Work out the finished part from the listing and answer in its coordinate system (mm). Face numbers are marked on the shaded views. A direction names the side the tool comes from. Round coordinates to 2 decimals unless told otherwise and drop trailing zeros. Loops run counter-clockwise (first coordinate to the right, second up) from the corner with the lowest first, then second, coordinate; pieces in that order, holes last.
Autodesk Inventor part; units mm, degrees
ref_plane "YZ Plane" through (0, 0, 0) normal (1, 0, 0) x (0, 1, 0)
ref_plane "XZ Plane" through (0, 0, 0) normal (0, 1, 0) x (-1, 0, 0)
ref_plane "XY Plane" through (0, 0, 0) normal (0, 0, 1) x (1, 0, 0)
sketch "Sketch1" plane through (0, 0, 0) normal (0, 1, 0) x (-1, 0, 0)
  line L0 (25, 25) -> (-25, 25)
  line L1 (-25, 25) -> (-25, -25)
  line L2 (-25, -25) -> (25, -25)
  line L3 (25, -25) -> (25, 25)
  line L4 (25, 25) -> (-25, -25) construction
  line L5 (-25, 25) -> (25, -25) construction
  point P0 (0, 0)
  dimension "d0" = 50
  dimension "d1" = 50
extrude "Extrusion1" add sketch "Sketch1" along normal blind 10
sketch "Sketch4" plane through (0, 10, 0) normal (0, 1, 0) x (1, 0, 0)
  circle A0 centre (0, 0) radius 25
  circle A1 centre (0, 0) radius 15
  dimension "d9" = 50
  dimension "d10" = 30
extrude "Extrusion3" add sketch "Sketch4" along normal blind 30
properties part number "Manipulator Base Type2"
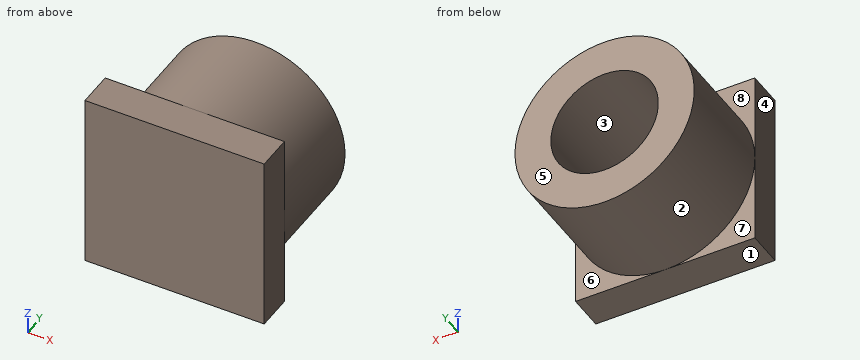
1. Find section B-B (x = 19). Write down the section's boundary in (y, z), then the cut area to 3 significant figures.
Answer key:
outline: (0, -25) - (10, -25) - (10, -16.25) - (40, -16.25) - (40, 16.25) - (10, 16.25) - (10, 25) - (0, 25) - close
area: 1,470 mm2
2. Consider probe 1 along X at (y, z) = (17, 0); probe 2 along Y at (x, z) = (-11.5, 0). Determine where each line is inside the solid, lowest interval first.
Answer key:
probe 1: x = -25 to -15, 15 to 25
probe 2: y = 0 to 10
3. Find section A-A (z = -20). Write down the section's boundary in (x, y), then the cut area to 3 significant figures.
Answer key:
outline: (-25, 0) - (25, 0) - (25, 10) - (15, 10) - (15, 40) - (-15, 40) - (-15, 10) - (-25, 10) - close
area: 1,400 mm2
4. Determine the mould class of the marked faces 1, 2, 3 and 4 for opening direction X: +X half, -X half, draft (parallel to the pull), parting line (faces both ways), or undercut.
Answer key:
face 1: draft
face 2: parting line
face 3: undercut
face 4: -X half
5. Find section C-C (y = 30). Write down the section's boundary in (x, z), then the cut area to 3 significant figures.
Answer key:
outline: circle Ø50 at (0, 0); hole circle Ø30 at (0, 0)
area: 1,260 mm2
6. Which of the six approach directions +Z, -Z, +X, -X, +Y, -Y give full straight-line access (tool end or side, diameter ignored) to the marked faces 5, 6, 7 and 8?
Answer key:
face 5: +Z, -Z, +X, -X, +Y
face 6: -Z, +X, +Y
face 7: -Z, -X, +Y
face 8: +Z, -X, +Y
7. Given pin 1 (5 mm diameter, centred on y = 23.5, z = 7, fed in from +X); pin 2 (6 mm diameter, centred on x = -4.5, z = 10.5, fed in from +Y); pin 3 (12 mm diameter, centred on y = 31.5, z = 18.5, fed in from -X), each flat-ended and moving along its own axis, determine where each tip first touches the part or whether it passes through.
Answer key:
pin 1: stops at x = 24.59
pin 2: stops at y = 10
pin 3: stops at x = -21.65
8. Find section D-D (z = 11.5). Write down the section's boundary in (x, y).
Answer key:
outline: (-25, 0) - (25, 0) - (25, 10) - (22.2, 10) - (22.2, 40) - (9.63, 40) - (9.63, 10) - (-9.63, 10) - (-9.63, 40) - (-22.2, 40) - (-22.2, 10) - (-25, 10) - close
